Can you work these out from the model? Positions are in its coordinate system, mm. A direction names the side the tool comes from. Coordinates: 2 decimals unless noted, no trailing zeros. Write each loop counter-clockwise with the first axis right and the second up, starting at its lowest first coordinate (ties: lowest second). Pieces come first, ordered by that corner, then holes.
Autodesk Inventor part; units mm, degrees
ref_plane "YZ Plane" through (0, 0, 0) normal (1, 0, 0) x (0, 1, 0)
ref_plane "XZ Plane" through (0, 0, 0) normal (0, 1, 0) x (-1, 0, 0)
ref_plane "XY Plane" through (0, 0, 0) normal (0, 0, 1) x (1, 0, 0)
sketch "Szkic1" plane through (0, 0, 0) normal (1, 0, 0) x (0, 1, 0)
  line L0 (0, -112) -> (0, 112) construction
  line L1 (-112, 0) -> (112, 0) construction
  circle A0 centre (0, 0) radius 67.6 construction
  line L2 (75.2, 7.6) -> (60, 7.6)
  line L3 (60, 7.6) -> (60, -7.6)
  line L4 (60, -7.6) -> (75.2, -7.6)
  line L5 (75.2, -7.6) -> (75.2, 7.6)
  line L6 (75.2, 7.6) -> (60, -7.6) construction
  line L7 (60, 7.6) -> (75.2, -7.6) construction
  circle A1 centre (0, 0) radius 80
  line L8 (61.3251, 44.1818) -> (48.1615, 36.5818)
  line L9 (48.1615, 36.5818) -> (55.7615, 23.4182)
  line L10 (55.7615, 23.4182) -> (68.9251, 31.0182)
  line L11 (68.9251, 31.0182) -> (61.3251, 44.1818)
  line L12 (61.3251, 44.1818) -> (55.7615, 23.4182) construction
  line L13 (48.1615, 36.5818) -> (68.9251, 31.0182) construction
  line L14 (31.0182, 68.9251) -> (23.4182, 55.7615)
  line L15 (23.4182, 55.7615) -> (36.5818, 48.1615)
  line L16 (36.5818, 48.1615) -> (44.1818, 61.3251)
  line L17 (44.1818, 61.3251) -> (31.0182, 68.9251)
  line L18 (31.0182, 68.9251) -> (36.5818, 48.1615) construction
  line L19 (23.4182, 55.7615) -> (44.1818, 61.3251) construction
  line L20 (-7.6, 75.2) -> (-7.6, 60)
  line L21 (-7.6, 60) -> (7.6, 60)
  line L22 (7.6, 60) -> (7.6, 75.2)
  line L23 (7.6, 75.2) -> (-7.6, 75.2)
  line L24 (-7.6, 75.2) -> (7.6, 60) construction
  line L25 (-7.6, 60) -> (7.6, 75.2) construction
  line L26 (-44.1818, 61.3251) -> (-36.5818, 48.1615)
  line L27 (-36.5818, 48.1615) -> (-23.4182, 55.7615)
  line L28 (-23.4182, 55.7615) -> (-31.0182, 68.9251)
  line L29 (-31.0182, 68.9251) -> (-44.1818, 61.3251)
  line L30 (-44.1818, 61.3251) -> (-23.4182, 55.7615) construction
  line L31 (-36.5818, 48.1615) -> (-31.0182, 68.9251) construction
  line L32 (-68.9251, 31.0182) -> (-55.7615, 23.4182)
  line L33 (-55.7615, 23.4182) -> (-48.1615, 36.5818)
  line L34 (-48.1615, 36.5818) -> (-61.3251, 44.1818)
  line L35 (-61.3251, 44.1818) -> (-68.9251, 31.0182)
  line L36 (-68.9251, 31.0182) -> (-48.1615, 36.5818) construction
  line L37 (-55.7615, 23.4182) -> (-61.3251, 44.1818) construction
  line L38 (-75.2, -7.6) -> (-60, -7.6) construction
  line L39 (-60, -7.6) -> (-60, 7.6) construction
  line L40 (-60, 7.6) -> (-75.2, 7.6) construction
  line L41 (-75.2, 7.6) -> (-75.2, -7.6) construction
  line L42 (-75.2, -7.6) -> (-60, 7.6) construction
  line L43 (-60, -7.6) -> (-75.2, 7.6) construction
  line L44 (-61.3251, -44.1818) -> (-48.1615, -36.5818)
  line L45 (-48.1615, -36.5818) -> (-55.7615, -23.4182)
  line L46 (-55.7615, -23.4182) -> (-68.9251, -31.0182)
  line L47 (-68.9251, -31.0182) -> (-61.3251, -44.1818)
  line L48 (-61.3251, -44.1818) -> (-55.7615, -23.4182) construction
  line L49 (-48.1615, -36.5818) -> (-68.9251, -31.0182) construction
  line L50 (-31.0182, -68.9251) -> (-23.4182, -55.7615)
  line L51 (-23.4182, -55.7615) -> (-36.5818, -48.1615)
  line L52 (-36.5818, -48.1615) -> (-44.1818, -61.3251)
  line L53 (-44.1818, -61.3251) -> (-31.0182, -68.9251)
  line L54 (-31.0182, -68.9251) -> (-36.5818, -48.1615) construction
  line L55 (-23.4182, -55.7615) -> (-44.1818, -61.3251) construction
  line L56 (7.6, -75.2) -> (7.6, -60)
  line L57 (7.6, -60) -> (-7.6, -60)
  line L58 (-7.6, -60) -> (-7.6, -75.2)
  line L59 (-7.6, -75.2) -> (7.6, -75.2)
  line L60 (7.6, -75.2) -> (-7.6, -60) construction
  line L61 (7.6, -60) -> (-7.6, -75.2) construction
  line L62 (44.1818, -61.3251) -> (36.5818, -48.1615)
  line L63 (36.5818, -48.1615) -> (23.4182, -55.7615)
  line L64 (23.4182, -55.7615) -> (31.0182, -68.9251)
  line L65 (31.0182, -68.9251) -> (44.1818, -61.3251)
  line L66 (44.1818, -61.3251) -> (23.4182, -55.7615) construction
  line L67 (36.5818, -48.1615) -> (31.0182, -68.9251) construction
  line L68 (68.9251, -31.0182) -> (55.7615, -23.4182)
  line L69 (55.7615, -23.4182) -> (48.1615, -36.5818)
  line L70 (48.1615, -36.5818) -> (61.3251, -44.1818)
  line L71 (61.3251, -44.1818) -> (68.9251, -31.0182)
  line L72 (68.9251, -31.0182) -> (48.1615, -36.5818) construction
  line L73 (55.7615, -23.4182) -> (61.3251, -44.1818) construction
  line L74 (0, 15.5) -> (-80, 15.5)
  line L75 (-80, 15.5) -> (-80, -15.5) construction
  line L76 (-80, -15.5) -> (0, -15.5)
  line L77 (0, -15.5) -> (0, 15.5)
  line L78 (0, 15.5) -> (-80, -15.5) construction
  line L79 (-80, 15.5) -> (0, -15.5) construction
  circle A2 centre (0, 0) radius 52
  line L80 (63.4, -5) -> (60.6, -5)
  line L81 (60.6, -5) -> (60.6, 5)
  line L82 (60.6, 5) -> (63.4, 5)
  line L83 (63.4, 5) -> (63.4, -5)
  line L84 (63.4, -5) -> (60.6, 5) construction
  line L85 (60.6, -5) -> (63.4, 5) construction
  line L86 (54.9811, 25.9699) -> (49.9811, 34.6301)
  line L87 (49.9811, 34.6301) -> (52.406, 36.0301)
  line L88 (52.406, 36.0301) -> (57.406, 27.3699)
  line L89 (57.406, 27.3699) -> (49.9811, 34.6301) construction
  line L90 (54.9811, 25.9699) -> (52.406, 36.0301) construction
  line L91 (57.406, 27.3699) -> (54.9811, 25.9699)
  line L92 (34.6301, 49.9811) -> (25.9699, 54.9811)
  line L93 (25.9699, 54.9811) -> (27.3699, 57.406)
  line L94 (27.3699, 57.406) -> (36.0301, 52.406)
  line L95 (36.0301, 52.406) -> (25.9699, 54.9811) construction
  line L96 (34.6301, 49.9811) -> (27.3699, 57.406) construction
  line L97 (36.0301, 52.406) -> (34.6301, 49.9811)
  line L98 (5, 60.6) -> (-5, 60.6)
  line L99 (-5, 60.6) -> (-5, 63.4)
  line L100 (-5, 63.4) -> (5, 63.4)
  line L101 (5, 63.4) -> (-5, 60.6) construction
  line L102 (5, 60.6) -> (-5, 63.4) construction
  line L103 (5, 63.4) -> (5, 60.6)
  line L104 (-25.9699, 54.9811) -> (-34.6301, 49.9811)
  line L105 (-34.6301, 49.9811) -> (-36.0301, 52.406)
  line L106 (-36.0301, 52.406) -> (-27.3699, 57.406)
  line L107 (-27.3699, 57.406) -> (-34.6301, 49.9811) construction
  line L108 (-25.9699, 54.9811) -> (-36.0301, 52.406) construction
  line L109 (-27.3699, 57.406) -> (-25.9699, 54.9811)
  line L110 (-49.9811, 34.6301) -> (-54.9811, 25.9699)
  line L111 (-54.9811, 25.9699) -> (-57.406, 27.3699)
  line L112 (-57.406, 27.3699) -> (-52.406, 36.0301)
  line L113 (-52.406, 36.0301) -> (-54.9811, 25.9699) construction
  line L114 (-49.9811, 34.6301) -> (-57.406, 27.3699) construction
  line L115 (-52.406, 36.0301) -> (-49.9811, 34.6301)
  line L116 (-60.6, 5) -> (-60.6, -5) construction
  line L117 (-60.6, -5) -> (-63.4, -5) construction
  line L118 (-63.4, -5) -> (-63.4, 5) construction
  line L119 (-63.4, 5) -> (-60.6, -5) construction
  line L120 (-60.6, 5) -> (-63.4, -5) construction
  line L121 (-63.4, 5) -> (-60.6, 5) construction
  line L122 (-54.9811, -25.9699) -> (-49.9811, -34.6301)
  line L123 (-49.9811, -34.6301) -> (-52.406, -36.0301)
  line L124 (-52.406, -36.0301) -> (-57.406, -27.3699)
  line L125 (-57.406, -27.3699) -> (-49.9811, -34.6301) construction
  line L126 (-54.9811, -25.9699) -> (-52.406, -36.0301) construction
  line L127 (-57.406, -27.3699) -> (-54.9811, -25.9699)
  line L128 (-34.6301, -49.9811) -> (-25.9699, -54.9811)
  line L129 (-25.9699, -54.9811) -> (-27.3699, -57.406)
  line L130 (-27.3699, -57.406) -> (-36.0301, -52.406)
  line L131 (-36.0301, -52.406) -> (-25.9699, -54.9811) construction
  line L132 (-34.6301, -49.9811) -> (-27.3699, -57.406) construction
  line L133 (-36.0301, -52.406) -> (-34.6301, -49.9811)
  line L134 (-5, -60.6) -> (5, -60.6)
  line L135 (5, -60.6) -> (5, -63.4)
  line L136 (5, -63.4) -> (-5, -63.4)
  line L137 (-5, -63.4) -> (5, -60.6) construction
  line L138 (-5, -60.6) -> (5, -63.4) construction
  line L139 (-5, -63.4) -> (-5, -60.6)
  line L140 (25.9699, -54.9811) -> (34.6301, -49.9811)
  line L141 (34.6301, -49.9811) -> (36.0301, -52.406)
  line L142 (36.0301, -52.406) -> (27.3699, -57.406)
  line L143 (27.3699, -57.406) -> (34.6301, -49.9811) construction
  line L144 (25.9699, -54.9811) -> (36.0301, -52.406) construction
  line L145 (27.3699, -57.406) -> (25.9699, -54.9811)
  line L146 (49.9811, -34.6301) -> (54.9811, -25.9699)
  line L147 (54.9811, -25.9699) -> (57.406, -27.3699)
  line L148 (57.406, -27.3699) -> (52.406, -36.0301)
  line L149 (52.406, -36.0301) -> (54.9811, -25.9699) construction
  line L150 (49.9811, -34.6301) -> (57.406, -27.3699) construction
  line L151 (52.406, -36.0301) -> (49.9811, -34.6301)
  circle A3 centre (-17, 65.4275) radius 2
  circle A4 centre (17, 65.4275) radius 2
  circle A5 centre (-17, -65.4275) radius 2
  circle A6 centre (17, -65.4275) radius 2
  point P0 (67.6, 0)
  point P1 (58.5433, 33.8)
  point P2 (33.8, 58.5433)
  point P3 (0, 67.6)
  point P4 (-33.8, 58.5433)
  point P5 (-58.5433, 33.8)
  point P6 (-67.6, 0)
  point P7 (-58.5433, -33.8)
  point P8 (-33.8, -58.5433)
  point P9 (0, -67.6)
  point P10 (33.8, -58.5433)
  point P11 (58.5433, -33.8)
  point P12 (-40, 0)
  point P13 (-49.6362, 15.5)
  point P14 (-49.6362, -15.5)
  point P15 (-78.4841, -15.5)
  point P16 (-78.4841, 15.5)
  point P17 (62, 0)
  point P18 (0, 0)
  point P19 (53.6936, 31)
  point P20 (31, 53.6936)
  point P21 (0, 62)
  point P22 (-31, 53.6936)
  point P23 (-53.6936, 31)
  point P24 (-62, 0)
  point P25 (-53.6936, -31)
  point P26 (-31, -53.6936)
  point P27 (0, -62)
  point P28 (31, -53.6936)
  point P29 (53.6936, -31)
  dimension "d1" = 15.2
  dimension "d2" = 15.2
  dimension "d3" = 160
  dimension "d6" = 360
  dimension "d8" = 60
  dimension "d13" = 31
  dimension "d14" = 104
  dimension "d15" = 2.8
  dimension "d16" = 10
  dimension "d17" = 62
  dimension "d20" = 360
  dimension "d22" = 4
  dimension "d23" = 17
extrude "Wyciągnięcie proste1" add sketch "Szkic1" against normal blind 7 contours L5 L4 L3 L2 | A1 L76 A2 L74 | L11 L10 L9 L8 | L17 L16 L15 L14 | L23 L22 L21 L20 | L29 L28 L27 L26 | L35 L34 L33 L32 | L47 L46 L45 L44 | L53 L52 L51 L50 | L59 L58 L57 L56 | L65 L64 L63 L62 | L71 L70 L69 L68 picked at (47.2911, 46.9149)
extrude "Wyciągnięcie proste2" cut sketch "Szkic1" against normal blind 2 contours L5 L4 L3 L2 | L11 L10 L9 L8 | L17 L16 L15 L14 | L23 L22 L21 L20 | L29 L28 L27 L26 | L35 L34 L33 L32 | L47 L46 L45 L44 | L53 L52 L51 L50 | L59 L58 L57 L56 | L65 L64 L63 L62 | L71 L70 L69 L68 | L80 L81 L82 L83 | L86 L87 L88 L91 | L92 L93 L94 L97 | L98 L99 L100 L103 | L104 L105 L106 L109 | L110 L111 L112 L115 | L122 L123 L124 L127 | L128 L129 L130 L133 | L134 L135 L136 L139 | L140 L141 L142 L145 | L146 L147 L148 L151
properties part number "uMule-podstawka_czujnikiIR"
1. I'm going to push flat-ended pins straight in: P1, Ø1.4, axis at x = -4.5, z = -62.5, coming from the -Y side; P2, Ø1.5, axis at x = -6, z = -11.5, coming from the -Y side; P3, Ø6, axis at y = 36.5, z = 62, coming from the +X side. Where does each tip first touch, or does it pass through?
2. If we section it at B-B, the plane y = 0: List the corners of the cut face in (x, z) for me.
3. We'd pull the mould along Y, two halves only. Please class faces 1 (the face through (-4.465, 30.239, -52.516)), 2 (the face through (-7, 52.5, 1.1)), 3 (the face through (-0.986, 27.165, -62.251)): released by +Y, released by -Y, zero draft, split by the parting line, or undercut.
4. If we section it at D-D, the plane x = -5.25: Count the separate pieces of the cut face and the enclosed holes in it, plus the area to 3 significant figures.
5. If we section it at A-A, the plane z = 0: List the corners of the cut face in (x, y) for me.
6. If I drill on L1, parallel to Z at x = -2.25, y = 0; L2, parallel to Y at x = -1.75, z = -55; L3, parallel to Z at x = -4.25, y = 17, over which ranges is the centre line in solid material (lowest first)?
7. If we section it at C-C, the plane y = -17: List the corners of the cut face in (x, z) for me.
8. Which directions (+Z, -Z, +X, -X, +Y, -Y) give clear straight access to the entire face, cutting with the end or side of a thin tool? Please do faces 4 (the face through (-4.465, -30.239, 52.516)), 5 (the face through (-0.986, 54.835, 40.435)).
Answers:
1. P1: stops at y = -50.8
1. P2: stops at y = 50.54
1. P3: stops at x = -2
2. outline: (-7, -80) - (0, -80) - (0, -75.2) - (-2, -75.2) - (-2, -63.4) - (-7, -63.4) - close; (-7, -60.6) - (-2, -60.6) - (-2, -60) - (0, -60) - (0, -52) - (-7, -52) - close; (-7, 52) - (0, 52) - (0, 60) - (-2, 60) - (-2, 60.6) - (-7, 60.6) - close; (-7, 63.4) - (-2, 63.4) - (-2, 75.2) - (0, 75.2) - (0, 80) - (-7, 80) - close
3. face 1: undercut
3. face 2: zero draft
3. face 3: undercut
4. separate pieces: 1
4. enclosed holes: 15
4. area: 10,400 mm2
5. outline: (-7, 52) - (0, 52) - (0, 60) - (-2, 60) - (-2, 60.6) - (-7, 60.6) - close; (-7, 63.4) - (-2, 63.4) - (-2, 75.2) - (0, 75.2) - (0, 80) - (-7, 80) - close
6. L1: z = -80 to -63.4, -60.6 to -52, 52 to 60.6, 63.4 to 80
6. L2: y = -58.09 to -40.53, -24.74 to 24.74, 40.53 to 58.09
6. L3: z = -78.17 to -67.43, -63.43 to -49.14, 49.14 to 63.43, 67.43 to 78.17
7. outline: (-7, -78.17) - (0, -78.17) - (0, -67.43) - (-7, -67.43) - close; (-7, -63.43) - (0, -63.43) - (0, -49.14) - (-7, -49.14) - close; (-7, 49.14) - (0, 49.14) - (0, 63.43) - (-7, 63.43) - close; (-7, 67.43) - (0, 67.43) - (0, 78.17) - (-7, 78.17) - close
8. face 4: +X, -X
8. face 5: +X
